Check sheet for the modelled part. Datum: model origin and axes. Units: mm. Face numbers are marked on the shaded views. Coordinates: 2 decimals unless noted, no trailing zeros. Order: outer loops, then holes, each group sorted by start corner. A loop starts at its lowest first (then second) coordinate and runs counter-clockwise, first axis right, second up.
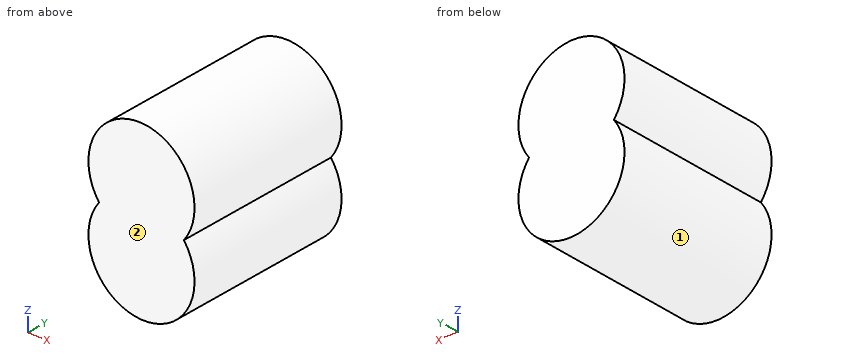
from build123d import *

# Parameters (mm, degrees)
F0_R      = 25
F1_DEPTH  = 75
F2_W      = 30.5
F2_H      = 30.5
F3_DEPTH  = 72
F4_R      = 25
F5_DEPTH  = 3
F6_R      = 25
F7_DEPTH  = 75
F8_W      = 30.5
F8_H      = 30.5
F9_DEPTH  = 72
F10_R     = 25
F11_DEPTH = 3


with BuildPart() as f1:
    # F0 (on Front) → F1 (new body)
    with BuildSketch(Plane.XZ):
        Circle(F0_R)
    extrude(amount=-F1_DEPTH)

    # F2 (on face) → F3 (cut, through all)
    with BuildSketch(Plane(origin=(0, 75, 0), x_dir=(-1, 0, 0), z_dir=(0, 1, 0))):
        Rectangle(F2_W, F2_H)
    extrude(amount=-F3_DEPTH, mode=Mode.SUBTRACT)

    # F4 (on face) → F5 (join)
    with BuildSketch(Plane(origin=(0, 75, 0), x_dir=(-1, 0, 0), z_dir=(0, 1, 0))):
        Circle(F4_R)
    extrude(amount=F5_DEPTH)

    # F6 (on Front) → F7 (join)
    with BuildSketch(Plane.XZ):
        with Locations((0, -30)):
            Circle(F6_R)
    extrude(amount=-F7_DEPTH)

    # F8 (on face) → F9 (cut, through all)
    with BuildSketch(Plane(origin=(0, 75, 0), x_dir=(-1, 0, 0), z_dir=(0, 1, 0))):
        with Locations((0, -30)):
            Rectangle(F8_W, F8_H)
    extrude(amount=-F9_DEPTH, mode=Mode.SUBTRACT)

    # F10 (on face) → F11 (join)
    with BuildSketch(Plane(origin=(0, 75, 0), x_dir=(-1, 0, 0), z_dir=(0, 1, 0))):
        with Locations((0, -30)):
            Circle(F10_R)
    extrude(amount=F11_DEPTH)


solid = f1.part
(1) Cross-section at C-C (z = -30). Enter the section's corners in (x, y), and give its area (3 significant figures).
Filled in:
outline: (-25, 0) - (25, 0) - (25, 78) - (-25, 78) - close; hole (-15.25, 3) - (15.25, 3) - (15.25, 75) - (-15.25, 75) - close
area: 1,700 mm2
(2) Cross-section at B-B (x = 0). Enter the section's corners in (y, z).
Filled in:
outline: (0, -55) - (78, -55) - (78, 25) - (0, 25) - close; hole (3, -45.25) - (75, -45.25) - (75, -14.75) - (3, -14.75) - close; hole (3, -5) - (75, -5) - (75, 15.25) - (3, 15.25) - close
(3) Go/stop test with flat-tipped pins: P1, Ø9, axis at y = 27, z = -33, coming from the -X side; P2, Ø8, axis at y = 61.5, z = -6.5, coming from the +X side; P3, Ø3, axis at x = -10.5, y = 45.5, coming from the -Z side. Record where each tip stops, or that it passes through.
Filled in:
P1: stops at x = -25
P2: stops at x = 24.87
P3: stops at z = -53.32
(4) Release check for a two-part mould opening along Z. For the marked faces 1 and 2 record: +Z half, -Z half, draft (parallel to the pull), parting line (faces both ways), or undercut.
Filled in:
face 1: undercut
face 2: draft
(5) Cross-section at D-D (z = -7.5). Enter the section's corners in (x, y).
Filled in:
outline: (-23.85, 0) - (23.85, 0) - (23.85, 78) - (-23.85, 78) - close; hole (-15.25, 3) - (-10.9, 3) - (-10.9, 75) - (-15.25, 75) - close; hole (10.9, 3) - (15.25, 3) - (15.25, 75) - (10.9, 75) - close
(6) Thickness scan on probe 1 along Y at (x, z) = (9.5, 4.5); probe 2 along Z at (x, y) = (2, 54); probe 3 along Z at (x, y) = (12, 7). Record the ranges inside material, lowest first.
Filled in:
probe 1: y = 0 to 3, 75 to 78
probe 2: z = -54.92 to -45.25, -14.75 to -5.08, 15.25 to 24.92
probe 3: z = -51.93 to -45.25, -14.75 to -8.07, 15.25 to 21.93
(7) Cross-section at A-A (y = 62). Enter the section's corners in (x, z), and give its area (3 significant figures).
Filled in:
outline: (-20, -15) arc R25 ccw (long way) to (20, -15) arc R25 ccw (long way) to start; hole (-15.25, -45.25) - (15.25, -45.25) - (15.25, -14.75) - (-15.25, -14.75) - close; hole (-15.25, -10.19) arc R25 cw to (15.25, -10.19) - (15.25, 15.25) - (-15.25, 15.25) - close
area: 1,770 mm2
